Can you work these out from the model? Positions are in its coordinate system, mm. Give positions to 0.01 mm unless a question says otherwise; leave off trailing zeros. Order: outer loops, then holes, each group sorted by start corner. A loop starts at its lowest first (then second) coordinate and runs counter-clockwise, first axis right, second up. Notation, with made-up numbers: M -33.75,9 L 7.25,9 A22 ccw 7.25,30 Z; hole C 80.25,39.5 d11. An arc over 180 degrees is marked long. Write each question's results on one line, items separated by ' | '.
from build123d import *

# Parameters (mm, degrees)
F0_W     = 32.258
F0_H     = 104.7641299665
F0_R     = 3.3734375
F0_R_2   = 9.779
F1_DEPTH = 6.35
F2_R     = 0.889
F3_DEPTH = 6.3914930276
F4_R     = 5.08
F5_SIZE  = 0.508


with BuildPart() as f1:
    # F0 (on Top) → F1 (new body)
    with BuildSketch(Plane.XY):
        with Locations((0, 0.4591811448)):
            Rectangle(F0_W, F0_H)
        with Locations((0, -37.4124510398)):
            Circle(F0_R, mode=Mode.SUBTRACT)
        Circle(F0_R_2, mode=Mode.SUBTRACT)
        with Locations((0, 38.3165156772)):
            Circle(F0_R, mode=Mode.SUBTRACT)
    extrude(amount=F1_DEPTH)

    # F2 (on face) → F3 (cut, through all)
    with BuildSketch(Plane(origin=(-16.129, 0, 0), x_dir=(0, -1, 0), z_dir=(-1, 0, 0))):
        with Locations((0, 3.175)):
            Circle(F2_R)
    extrude(amount=-F3_DEPTH, mode=Mode.SUBTRACT)

    # F4
    f4_edges = [f1.edges().sort_by_distance(p)[0] for p in [
        (-16.129, 52.841246, 3.175),
        (-16.129, -51.922884, 3.175),
        (16.129, -51.922884, 3.175),
        (16.129, 52.841246, 3.175),
    ]]
    fillet(f4_edges, radius=F4_R)

    # F5
    f5_edges = [f1.edges().sort_by_distance(p)[0] for p in [
        (-3.373437, 38.316516, 6.35),
        (-3.373437, 38.316516, 0),
        (-9.779, 0, 0),
        (-3.373437, -37.412451, 0),
        (-3.373437, -37.412451, 6.35),
        (-9.779, 0, 6.35),
    ]]
    chamfer(f5_edges, length=F5_SIZE)


solid = f1.part
(1) Imagine slicing it at B-B, the plane x = 0. Write out the boundary of the cut face in (y, z).
Data:
outline: M -51.92,0 L -41.29,0 L -40.79,0.51 L -40.79,5.84 L -41.29,6.35 L -51.92,6.35 Z; M -34.04,0.51 L -33.53,0 L -10.29,0 L -9.78,0.51 L -9.78,5.84 L -10.29,6.35 L -33.53,6.35 L -34.04,5.84 Z; M 9.78,0.51 L 10.29,0 L 34.44,0 L 34.94,0.51 L 34.94,5.84 L 34.44,6.35 L 10.29,6.35 L 9.78,5.84 Z; M 41.69,0.51 L 42.2,0 L 52.84,0 L 52.84,6.35 L 42.2,6.35 L 41.69,5.84 Z
(2) We'd pull the mould along Z, two halves only. Please class faces 1 (the face through (-12.978, -0.478, 3.925)), 2 (the face through (-11, 1, 0)), 3 (the face through (14.601, -50.474, 3.219)): +Z half, -Z half, draft (parallel to the pull), parting line (faces both ways), or undercut.
Data:
face 1: undercut | face 2: -Z half | face 3: draft
(3) I need wall thicknesses on L1, parallel to Y at x = 0, z = 2.3; L2, parallel to X at y = 0, z = 4.25; L3, parallel to Y at x = -1, z = 3.5. Which ranges of each line are inside material? Lowest first, please. Write a range as from..to.
Data:
L1: y = -51.92..-40.79, -34.04..-9.78, 9.78..34.94, 41.69..52.84 | L2: x = -16.13..-9.78, 9.78..16.13 | L3: y = -51.92..-40.63, -34.19..-9.73, 9.73..35.09, 41.54..52.84
(4) Imagine slicing it at A-A, the plane y = 0. Write out the boundary of the cut face in (x, z), plus the area to 3 significant figures.
Data:
outline: M -16.13,0 L -10.29,0 L -9.78,0.51 L -9.78,2.29 L -16.13,2.29 Z; M -16.13,4.06 L -9.78,4.06 L -9.78,5.84 L -10.29,6.35 L -16.13,6.35 Z; M 9.78,0.51 L 10.29,0 L 16.13,0 L 16.13,6.35 L 10.29,6.35 L 9.78,5.84 Z | area: 68.8 mm2
(5) Will this pin go through, and if not, where does the flat tip stop? P1, Ø5.5, axis at x = 0, y = -37.41, coming from the -Z side (3 decimals).
Data:
P1: passes through
